from build123d import *

# Parameters (mm, degrees)
SKETCH_1_W      = 10
SKETCH_1_H      = 44
SKETCH_1_R      = 1.15
EXTRUDE_1_DEPTH = 4
SKETCH_2_R      = 2.25
SKETCH_2_R_2    = 1.15
EXTRUDE_2_DEPTH = 3


with BuildPart() as part:
    # 草图1 → 凸台-拉伸1 (new body)
    with BuildSketch(Plane(origin=(0, 0, 0), x_dir=(1, 0, 0), z_dir=(0, 1, 0))):
        Rectangle(SKETCH_1_W, SKETCH_1_H)
        with Locations(Location((0, -18, 0), (0, 0, 270))):
            Circle(SKETCH_1_R, mode=Mode.SUBTRACT)
        with Locations(Location((0, 18, 0), (0, 0, 270))):
            Circle(SKETCH_1_R, mode=Mode.SUBTRACT)
    extrude(amount=EXTRUDE_1_DEPTH)

    # 草图2 → 凸台-拉伸2 (add)
    # profile 1 of 3: a face of its own
    with BuildSketch(Plane(origin=(0, 4, 0), x_dir=(1, 0, 0), z_dir=(0, 1, 0))):
        Polygon((-5, 32), (-5, 22), (5, 22), (5, 32), (5, 46.5), (24.5, 46.5), (24.5, 53), (-5, 53), (-5, 45.896329407), align=None)
        with Locations(Location((18, 49.5, 0), (0, 0, 270))):
            Circle(SKETCH_2_R, mode=Mode.SUBTRACT)
    # profile 2 of 3: a face of its own
    with BuildSketch(Plane(origin=(0, 4, 0), x_dir=(1, 0, 0), z_dir=(0, 1, 0))):
        Polygon((-5, -12), (-5, -22), (5, -22), (5, -12), (5, 22), (-5, 22), align=None)
        with Locations(Location((0, -18, 0), (0, 0, 270))):
            Circle(SKETCH_2_R_2, mode=Mode.SUBTRACT)
        with Locations(Location((0, 18, 0), (0, 0, 270))):
            Circle(SKETCH_2_R_2, mode=Mode.SUBTRACT)
    # profile 3 of 3: a face of its own
    with BuildSketch(Plane(origin=(0, 4, 0), x_dir=(1, 0, 0), z_dir=(0, 1, 0))):
        Polygon((24.5, -36.5), (5, -36.5), (5, -22), (-5, -22), (-5, -43), (24.5, -43), align=None)
        with Locations(Location((18, -39.5, 0), (0, 0, 270))):
            Circle(SKETCH_2_R, mode=Mode.SUBTRACT)
    extrude(amount=EXTRUDE_2_DEPTH)


solid = part.part
Verification items for the finished model (mm, model axes). A direction names the side the tool comes from. Coordinates: 2 decimals unless noted, no trailing zeros. Order: outer loops, then holes, each group sorted by start corner. A loop starts at its lowest first (then second) coordinate and runs counter-clockwise, first axis right, second up. Notation, with made-up numbers: M 65.25,78.5 L 94.25,78.5 A29 cw 94.25,104.5 Z; hole C 44,-2.5 d2. An arc over 180 degrees is marked long. One line per item, written item: value. Start each with the question number.
Item 1: Sectioned sample at D-D on x = 9. Record the cut outline in (y, z).
Item 2: Thickness scan on probe 1 along Z at (x, y) = (12.25, 5.5); probe 2 along X at (y, z) = (4.5, 18); probe 3 along X at (y, z) = (5, 39.5). Record the ranges inside material, lowest first.
Item 3: Sectioned sample at C-C on z = -18. Record the cut outline in (x, y), then the cut area to 3 significant figures.
Item 4: Sectioned sample at A-A on x = 0. Record the cut outline in (y, z), then the cut area to 3 significant figures.
Item 5: Sectioned sample at B-B on x = 18. Record the cut outline in (y, z), then the cut area to 3 significant figures.
Item 6: Mould release check, pull along X, two halves, no side actions. Record for faces 1 (the flat face through (-5, 4, -6)), 2 (the flat face through (24.5, 5, -50)), 3 (the flat face through (3, 4, 35)), 4 (the cylindrical face through (16.631, 5.479, -51.286)): pulls with the +X half, pulls with the -X half, needs draft (parallel to the pull), parting line crosses it, or undercut.
Item 7: Depth check by flat-ended pin: P1, Ø2, axis at y = 2.5, z = 15.5, coming from the +X side; P2, Ø8, axis at x = 1.5, z = -26.5, coming from the -Y side; P3, Ø1.2, axis at x = 2.5, y = 1.5, coming from the -Z side. Enter the tip coordinate at first touch or a pass-through.
Item 8: Access from +Z, -Z, +X, -X, +Y, -Y to the whole of each face (thin tool, end or side, straight path). Record for faces 5 (the flat face through (0, 2, 22)), 6 (the flat face through (0, 2, -22)), 7 (the flat face through (15, 5, 36.5)).
Calculated:
1. outline: M 4,-53 L 7,-53 L 7,-46.5 L 4,-46.5 Z; M 4,36.5 L 7,36.5 L 7,43 L 4,43 Z
2. probe 1: -53 to -46.5, 36.5 to 43
2. probe 2: -5 to -1.15, 1.15 to 5
2. probe 3: -5 to 15.75, 20.25 to 24.5
3. outline: M -5,0 L -1.15,0 L -1.15,7 L -5,7 Z; M 1.15,0 L 5,0 L 5,7 L 1.15,7 Z
3. area: 53.9 mm^2
4. outline: M 0,-22 L 4,-22 L 4,-53 L 7,-53 L 7,-19.15 L 0,-19.15 Z; M 0,-16.85 L 7,-16.85 L 7,16.85 L 0,16.85 Z; M 0,19.15 L 7,19.15 L 7,43 L 4,43 L 4,22 L 0,22 Z
4. area: 432 mm^2
5. outline: M 4,-53 L 7,-53 L 7,-51.75 L 4,-51.75 Z; M 4,-47.25 L 7,-47.25 L 7,-46.5 L 4,-46.5 Z; M 4,36.5 L 7,36.5 L 7,37.25 L 4,37.25 Z; M 4,41.75 L 7,41.75 L 7,43 L 4,43 Z
5. area: 12.0 mm^2
6. face 1: pulls with the -X half
6. face 2: pulls with the +X half
6. face 3: needs draft
6. face 4: undercut
7. P1: x = 5
7. P2: y = 4
7. P3: z = -22
8. face 5: +Z, +X, -X, -Y
8. face 6: -Z, +X, -X, -Y
8. face 7: +X, +Y, -Y
